Part model, mm, in its own coordinate system. A direction names the side the tool comes from. Round coordinates to 2 decimals unless told otherwise and drop trailing zeros. Loops run counter-clockwise (first coordinate to the right, second up) from the corner with the lowest first, then second, coordinate; pieces in that order, holes last.
from build123d import *

# Parameters (mm, degrees)
SKETCH_1_R      = 3.9
SKETCH_1_R_2    = 3.4
EXTRUDE_1_DEPTH = 100


with BuildPart() as part:
    # 草图1 → 凸台-拉伸1 (new body)
    with BuildSketch(Plane.XY):
        Polygon((-23.218782805, 39.545792426), (-38.968782805, 39.545792426), (-38.968782805, 23.795792426), (-35.968782805, 23.795792426), (-35.968782805, 26.745792426), (-27.968782805, 26.745792426), (-27.968782805, 23.795792426), (-24.968782805, 23.795792426), (-24.968782805, 15.295792426), (-27.968782805, 15.295792426), (-27.968782805, 12.345792426), (-35.968782805, 12.345792426), (-35.968782805, 15.295792426), (-38.968782805, 15.295792426), (-38.968782805, -0.454207574), (-38.968782805, -16.204207574), (-35.968782805, -16.204207574), (-35.968782805, -13.254207574), (-27.968782805, -13.254207574), (-27.968782805, -16.204207574), (-24.968782805, -16.204207574), (-24.968782805, -24.704207574), (-27.968782805, -24.704207574), (-27.968782805, -27.654207574), (-35.968782805, -27.654207574), (-35.968782805, -24.704207574), (-38.968782805, -24.704207574), (-38.968782805, -40.454207574), (-23.218782805, -40.454207574), (-23.218782805, -37.454207574), (-26.168782805, -37.454207574), (-26.168782805, -29.454207574), (-23.218782805, -29.454207574), (-23.218782805, -26.454207574), (-14.718782805, -26.454207574), (-14.718782805, -29.454207574), (-11.768782805, -29.454207574), (-11.768782805, -37.454207574), (-14.718782805, -37.454207574), (-14.718782805, -40.454207574), (1.031217195, -40.454207574), (16.781217195, -40.454207574), (16.781217195, -37.454207574), (13.831217195, -37.454207574), (13.831217195, -29.454207574), (16.781217195, -29.454207574), (16.781217195, -26.454207574), (25.281217195, -26.454207574), (25.281217195, -29.454207574), (28.231217195, -29.454207574), (28.231217195, -37.454207574), (25.281217195, -37.454207574), (25.281217195, -40.454207574), (41.031217195, -40.454207574), (41.031217195, -24.704207574), (38.031217195, -24.704207574), (38.031217195, -27.654207574), (30.031217195, -27.654207574), (30.031217195, -24.704207574), (27.031217195, -24.704207574), (27.031217195, -16.204207574), (30.031217195, -16.204207574), (30.031217195, -13.254207574), (38.031217195, -13.254207574), (38.031217195, -16.204207574), (41.031217195, -16.204207574), (41.031217195, -0.454207574), (41.031217195, 15.295792426), (38.031217195, 15.295792426), (38.031217195, 12.345792426), (30.031217195, 12.345792426), (30.031217195, 15.295792426), (27.031217195, 15.295792426), (27.031217195, 23.795792426), (30.031217195, 23.795792426), (30.031217195, 26.745792426), (38.031217195, 26.745792426), (38.031217195, 23.795792426), (41.031217195, 23.795792426), (41.031217195, 39.545792426), (25.281217195, 39.545792426), (25.281217195, 36.545792426), (28.231217195, 36.545792426), (28.231217195, 28.545792426), (25.281217195, 28.545792426), (25.281217195, 25.545792426), (16.781217195, 25.545792426), (16.781217195, 28.545792426), (13.831217195, 28.545792426), (13.831217195, 36.545792426), (16.781217195, 36.545792426), (16.781217195, 39.545792426), (1.031217195, 39.545792426), (-14.718782805, 39.545792426), (-14.718782805, 36.545792426), (-11.768782805, 36.545792426), (-11.768782805, 28.545792426), (-14.718782805, 28.545792426), (-14.718782805, 25.545792426), (-23.218782805, 25.545792426), (-23.218782805, 28.545792426), (-26.168782805, 28.545792426), (-26.168782805, 36.545792426), (-23.218782805, 36.545792426), align=None)
        with Locations((-32.568782805, 33.145792426)):
            Circle(SKETCH_1_R, mode=Mode.SUBTRACT)
        with Locations((-18.968782805, 19.545792426)):
            Circle(SKETCH_1_R_2, mode=Mode.SUBTRACT)
        with Locations((34.631217195, 33.145792426)):
            Circle(SKETCH_1_R, mode=Mode.SUBTRACT)
        with Locations((21.031217195, 19.545792426)):
            Circle(SKETCH_1_R_2, mode=Mode.SUBTRACT)
        with Locations((-32.568782805, -34.054207574)):
            Circle(SKETCH_1_R, mode=Mode.SUBTRACT)
        with Locations((-18.968782805, -20.454207574)):
            Circle(SKETCH_1_R_2, mode=Mode.SUBTRACT)
        with Locations((34.631217195, -34.054207574)):
            Circle(SKETCH_1_R, mode=Mode.SUBTRACT)
        with Locations((21.031217195, -20.454207574)):
            Circle(SKETCH_1_R_2, mode=Mode.SUBTRACT)
        Polygon((-23.218782805, 13.545792426), (-14.718782805, 13.545792426), (-14.718782805, 15.295792426), (-12.968782805, 15.295792426), (-12.968782805, 23.795792426), (-8.768782805, 28.545792426), (-8.768782805, 34.545792426), (10.831217195, 34.545792426), (10.831217195, 28.545792426), (15.031217195, 23.795792426), (15.031217195, 15.295792426), (16.781217195, 15.295792426), (16.781217195, 13.545792426), (25.281217195, 13.545792426), (30.031217195, 9.345792426), (36.031217195, 9.345792426), (36.031217195, -10.254207574), (30.031217195, -10.254207574), (25.281217195, -14.454207574), (16.781217195, -14.454207574), (16.781217195, -16.204207574), (15.031217195, -16.204207574), (15.031217195, -24.704207574), (10.831217195, -29.454207574), (10.831217195, -35.454207574), (-8.768782805, -35.454207574), (-8.768782805, -29.454207574), (-12.968782805, -24.704207574), (-12.968782805, -16.204207574), (-14.718782805, -16.204207574), (-14.718782805, -14.454207574), (-23.218782805, -14.454207574), (-27.968782805, -10.254207574), (-33.968782805, -10.254207574), (-33.968782805, 9.345792426), (-27.968782805, 9.345792426), align=None, mode=Mode.SUBTRACT)
    extrude(amount=EXTRUDE_1_DEPTH)


solid = part.part
1) Drop flat-ended pins along their axis: pin 1 Ø10 at (x, y) = (-16, 5) entering from -Z; pin 2 Ø3 at (y, z) = (-22.5, 34) entering from -X; pin 3 Ø3 at (x, z) = (-17, 67.5) entering from +Y. Give the stop position or say it passes through.
Values:
pin 1: passes through
pin 2: stops at x = -24.97
pin 3: stops at y = 25.55
2) Slice it at A-A, the plane x = 8. Give the cut face in (y, z), then the cut area to 3 significant figures.
Values:
outline: (-40.45, 0) - (-35.45, 0) - (-35.45, 100) - (-40.45, 100) - close; (34.55, 0) - (39.55, 0) - (39.55, 100) - (34.55, 100) - close
area: 1,000 mm2
3) Tool access for faces 1 (the face through (40, -16.204, 49)), 2 (the face through (33, 9.346, 49)), 3 (the face through (-19, -26.454, 49)), 4 (the face through (-24.969, -20, 49)): list every direction of +Z, -Z, +X, -X, +Y, -Y with a clear straight run to the whole face (end or side of a thin tool).
Values:
face 1: +Z, -Z, +X
face 2: +Z, -Z
face 3: +Z, -Z, -Y
face 4: +Z, -Z, -X
4) Mould opens along X. For faces 5 (the face through (-23.219, -28, 49)), 6 (the face through (15.031, -20, 49)), 7 (the face through (-38.969, -32, 49)), 8 (the face through (41.031, -1, 49)) say: released by +X, released by -X, zero draft, split by the parting line, or undercut.
Values:
face 5: undercut
face 6: undercut
face 7: released by -X
face 8: released by +X
5) Slice it at C-C, the plane z = 92. Give the number of separate pieces and of enclosed holes in the cut face, then the cut area to 3 significant figures.
Values:
separate pieces: 1
enclosed holes: 9
area: 1,870 mm2
6) Slice it at B-B, the plane x = 20. Give the cut face in (y, z), then the cut area to 3 significant figures.
Values:
outline: (-26.45, 0) - (-23.69, 0) - (-23.69, 100) - (-26.45, 100) - close; (-17.21, 0) - (-14.45, 0) - (-14.45, 100) - (-17.21, 100) - close; (13.55, 0) - (16.31, 0) - (16.31, 100) - (13.55, 100) - close; (22.79, 0) - (25.55, 0) - (25.55, 100) - (22.79, 100) - close
area: 1,100 mm2
7) Wall check: line 1 along X through (y, z) = (-14.5, 20); line 2 along X through (y, z) = (-34, 50); line 3 along Y through (x, z) = (-14, 17). Give the ranges that are in metal, low to high.
Values:
line 1: x = -38.97 to -35.97, -27.97 to -14.72, 16.78 to 30.03, 38.03 to 41.03
line 2: x = -38.97 to -36.47, -28.67 to -26.17, -11.77 to -8.77, 10.83 to 13.83, 28.23 to 30.73, 38.53 to 41.03
line 3: y = -40.45 to -37.45, -29.45 to -16.2, 15.3 to 28.55, 36.55 to 39.55
